Geometry: final body of the model. Coordinates: model frame, mm. A direction names the side the tool comes from. Round coordinates to 2 decimals unless told otherwise and drop trailing zeros. Order: outer loops, then holes, each group sorted by start corner. A loop starts at its lowest first (then second) coordinate and runs counter-clockwise, first axis right, second up. Notation, with made-up numbers: M 31.5,18.5 L 55.5,18.5 A7 cw 55.5,31.5 Z; hole C 68,45 d10. An arc over 180 degrees is marked long. Return JSON: item names as keys, results as strings. Group by question number.
Q1. Access query for faces 5 (the face through (-5, 10, 15)), 6 (the face through (60, 8, 87)), 7 (the face through (44, 0, 44)), 8 (the face through (6, 21, 42)). Directions: +Z, -Z, +X, -X, +Y, -Y. A direction counts if a zero-diameter tool reaches every point of the face in a straight line with its end or side. Return the directions, or none.
Q2. Contact query for flat-ended pins moving along their axis: pin 1 (1 mm diameter, centred on y = 23.5, z = 31, fed in from -X); pin 2 (4 mm diameter, centred on y = 15.5, z = 76.5, fed in from +X); pin 3 (5 mm diameter, centred on x = 57.5, y = 6.5, fed in from -Z). Output: stop coordinate, or through.
Q3. Cut plane D-D on x = -4. Output: boundary loops of the cut face in (y, z), and give its area (3 significant figures).
Q4. Cut plane C-C on x = 20.32. Output: boundary loops of the cut face in (y, z), and give its area (3 significant figures).
Q5. Mould query, pull axis X, two halves, no side actions, for faces 1 (the face through (72.45, 23.36, 87.46)), 2 (the face through (44, 30, 44)), 3 (the face through (101, 10, 7)), 4 (the face through (87, 26, 42)). Classes: released by +X, released by -X, zero draft, split by the parting line, or undercut.
Q6. Cut plane B-B on y = 13. Output: boundary loops of the cut face in (x, z), and give its area (3 significant figures).
Q7. Ray query, probe 1 along X at (y, z) = (22, 77); probe 2 along Y at (x, z) = (58, 47); probe 3 along Y at (x, z) = (69.68, 88). Return the intervals inside material, ascending.
Q8. Cut plane A-A on x = 52.5. Output: boundary loops of the cut face in (y, z), and give its area (3 significant figures).
```python
from build123d import *

# Parameters (mm, degrees)
SKETCH1_W           = 90
SKETCH1_H           = 30
BOSS_EXTRUDE1_DEPTH = 90
SKETCH2_W           = 84
SKETCH2_H           = 4
CUT_EXTRUDE1_DEPTH  = 85
SKETCH3_W           = 74
SKETCH3_H           = 3
CUT_EXTRUDE2_DEPTH  = 85
SKETCH4_W           = 84
SKETCH4_H           = 3
CUT_EXTRUDE3_DEPTH  = 85
SKETCH5_W           = 74
SKETCH5_H           = 3
CUT_EXTRUDE4_DEPTH  = 85
SKETCH7_W           = 84
SKETCH7_H           = 4
CUT_EXTRUDE5_DEPTH  = 85
SKETCH8_W           = 74
SKETCH8_H           = 3
CUT_EXTRUDE6_DEPTH  = 85
SKETCH9_W           = 84
SKETCH9_H           = 3
CUT_EXTRUDE7_DEPTH  = 85
SKETCH10_W          = 74
SKETCH10_H          = 3
CUT_EXTRUDE8_DEPTH  = 85
SKETCH11_R          = 3
CUT_EXTRUDE9_DEPTH  = 85
SKETCH12_W          = 30
SKETCH12_H          = 3
CUT_EXTRUDE10_DEPTH = 85
SKETCH13_W          = 15
SKETCH13_H          = 20
BOSS_EXTRUDE2_DEPTH = 11
SKETCH14_R          = 5
CUT_EXTRUDE11_DEPTH = 10


with BuildPart() as part:
    # Sketch1 → Boss-Extrude1 (new body)
    with BuildSketch(Plane.XY):
        with Locations((45, 15)):
            Rectangle(SKETCH1_W, SKETCH1_H)
    extrude(amount=BOSS_EXTRUDE1_DEPTH)

    # Sketch2 → Cut-Extrude1 (cut)
    with BuildSketch(Plane(origin=(0, 0, 0), x_dir=(-1, 0, 0), z_dir=(0, 0, -1))):
        with Locations((-45, 26)):
            Rectangle(SKETCH2_W, SKETCH2_H)
    extrude(amount=-CUT_EXTRUDE1_DEPTH, mode=Mode.SUBTRACT)

    # Sketch3 → Cut-Extrude2 (cut)
    with BuildSketch(Plane(origin=(0, 0, 0), x_dir=(-1, 0, 0), z_dir=(0, 0, -1))):
        with Locations((-45, 22.5)):
            Rectangle(SKETCH3_W, SKETCH3_H)
    extrude(amount=-CUT_EXTRUDE2_DEPTH, mode=Mode.SUBTRACT)

    # Sketch4 → Cut-Extrude3 (cut)
    with BuildSketch(Plane(origin=(0, 0, 0), x_dir=(-1, 0, 0), z_dir=(0, 0, -1))):
        with Locations((-45, 19.5)):
            Rectangle(SKETCH4_W, SKETCH4_H)
    extrude(amount=-CUT_EXTRUDE3_DEPTH, mode=Mode.SUBTRACT)

    # Sketch5 → Cut-Extrude4 (cut)
    with BuildSketch(Plane(origin=(0, 0, 0), x_dir=(-1, 0, 0), z_dir=(0, 0, -1))):
        with Locations((-45, 16.5)):
            Rectangle(SKETCH5_W, SKETCH5_H)
    extrude(amount=-CUT_EXTRUDE4_DEPTH, mode=Mode.SUBTRACT)

    # Sketch7 → Cut-Extrude5 (cut)
    with BuildSketch(Plane(origin=(0, 0, 0), x_dir=(-1, 0, 0), z_dir=(0, 0, -1))):
        with Locations((-45, 13)):
            Rectangle(SKETCH7_W, SKETCH7_H)
    extrude(amount=-CUT_EXTRUDE5_DEPTH, mode=Mode.SUBTRACT)

    # Sketch8 → Cut-Extrude6 (cut)
    with BuildSketch(Plane(origin=(0, 0, 0), x_dir=(-1, 0, 0), z_dir=(0, 0, -1))):
        with Locations((-45, 9.5)):
            Rectangle(SKETCH8_W, SKETCH8_H)
    extrude(amount=-CUT_EXTRUDE6_DEPTH, mode=Mode.SUBTRACT)

    # Sketch9 → Cut-Extrude7 (cut)
    with BuildSketch(Plane(origin=(0, 0, 0), x_dir=(-1, 0, 0), z_dir=(0, 0, -1))):
        with Locations((-45, 6.5)):
            Rectangle(SKETCH9_W, SKETCH9_H)
    extrude(amount=-CUT_EXTRUDE7_DEPTH, mode=Mode.SUBTRACT)

    # Sketch10 → Cut-Extrude8 (cut)
    with BuildSketch(Plane(origin=(0, 0, 0), x_dir=(-1, 0, 0), z_dir=(0, 0, -1))):
        with Locations((-45, 3.5)):
            Rectangle(SKETCH10_W, SKETCH10_H)
    extrude(amount=-CUT_EXTRUDE8_DEPTH, mode=Mode.SUBTRACT)

    # Sketch11 → Cut-Extrude9 (cut)
    with BuildSketch(Plane(origin=(0, 0, 85), x_dir=(-1, 0, 0), z_dir=(0, 0, -1))):
        with Locations((-20.32, 24.51)):
            Circle(SKETCH11_R)
    cut_extrude9 = extrude(amount=-CUT_EXTRUDE9_DEPTH, mode=Mode.SUBTRACT)

    # Mirror1: Cut-Extrude9 across plane
    add(cut_extrude9.mirror(Plane.ZY.offset(-45)), mode=Mode.SUBTRACT)

    # Sketch12 → Cut-Extrude10 (cut)
    with BuildSketch(Plane(origin=(0, 0, 85), x_dir=(-1, 0, 0), z_dir=(0, 0, -1))):
        with Locations((-45, 22.5)):
            Rectangle(SKETCH12_W, SKETCH12_H)
    cut_extrude10 = extrude(amount=-CUT_EXTRUDE10_DEPTH, mode=Mode.SUBTRACT)

    # Mirror2: Cut-Extrude10 across plane
    add(cut_extrude10.mirror(Plane.ZX.offset(15)), mode=Mode.SUBTRACT)

    # Sketch13 → Boss-Extrude2 (add)
    with BuildSketch(Plane.ZY):
        with Locations((7.5, 10)):
            Rectangle(SKETCH13_W, SKETCH13_H)
    boss_extrude2 = extrude(amount=BOSS_EXTRUDE2_DEPTH)

    # Mirror3: Boss-Extrude2 across plane
    add(boss_extrude2.mirror(Plane.ZY.offset(-45)))

    # Sketch14 → Cut-Extrude11 (cut)
    with BuildSketch(Plane(origin=(0, 0, 0), x_dir=(-1, 0, 0), z_dir=(0, 0, -1))):
        with Locations((4, 10)):
            Circle(SKETCH14_R)
    cut_extrude11 = extrude(amount=-CUT_EXTRUDE11_DEPTH, mode=Mode.SUBTRACT)

    # Mirror4: Cut-Extrude11 across plane
    add(cut_extrude11.mirror(Plane.ZY.offset(-45)), mode=Mode.SUBTRACT)


solid = part.part
```
Result sheet:
{
 "1": {"face 5": "+Z, -X, +Y, -Y", "face 6": "+Z, -Z", "face 7": "+Z, -Z, +X, -X, -Y", "face 8": "-Z"},
 "2": {"pin 1": "stops at x = 0", "pin 2": "stops at x = 90", "pin 3": "stops at z = 85"},
 "3": {"outline": "M 0,0 L 5,0 L 5,10 L 15,10 L 15,0 L 20,0 L 20,15 L 0,15 Z", "area": "200 mm²"},
 "4": {"outline": "M 0,0 L 2,0 L 2,85 L 21.51,85 L 21.51,90 L 0,90 Z; M 27.51,85 L 28,85 L 28,0 L 30,0 L 30,90 L 27.51,90 Z", "area": "460 mm²"},
 "5": {"face 1": "undercut", "face 2": "zero draft", "face 3": "released by +X", "face 4": "undercut"},
 "6": {"outline": "M -11,0 L -8,0 L -8,10 L 0,10 L 0,0 L 3,0 L 3,85 L 87,85 L 87,0 L 90,0 L 90,10 L 98,10 L 98,0 L 101,0 L 101,15 L 90,15 L 90,90 L 0,90 L 0,15 L -11,15 Z", "area": "1,130 mm²"},
 "7": {"probe 1": "x = 0 to 8, 82 to 90", "probe 2": "y = 0 to 2, 28 to 30", "probe 3": "y = 0 to 21.51, 27.51 to 30"},
 "8": {"outline": "M 0,0 L 2,0 L 2,85 L 6,85 L 6,90 L 0,90 Z; M 9,85 L 21,85 L 21,90 L 9,90 Z; M 24,85 L 28,85 L 28,0 L 30,0 L 30,90 L 24,90 Z", "area": "460 mm²"}
}
